```python
from build123d import *

# Parameters (mm, degrees)
SKETCH1_W           = 50
SKETCH1_H           = 50
BOSS_EXTRUDE1_DEPTH = 5
SKETCH2_W           = 50
SKETCH2_H           = 5
BOSS_EXTRUDE2_DEPTH = 50
SKETCH3_R           = 2.6
CUT_EXTRUDE1_DEPTH  = 50
CHAMFER1_SIZE       = 20
SKETCH4_R           = 2.6
CUT_EXTRUDE2_DEPTH  = 50
CHAMFER2_SIZE       = 20
CHAMFER3_SIZE       = 2
CHAMFER4_SIZE       = 2


with BuildPart() as part:
    # Sketch1 → Boss-Extrude1 (new body)
    with BuildSketch(Plane(origin=(0, 0, 0), x_dir=(1, 0, 0), z_dir=(0, 1, 0))):
        Rectangle(SKETCH1_W, SKETCH1_H)
    extrude(amount=BOSS_EXTRUDE1_DEPTH)

    # Sketch2 → Boss-Extrude2 (add)
    with BuildSketch(Plane(origin=(0, 5, 0), x_dir=(1, 0, 0), z_dir=(0, 1, 0))):
        with Locations((0, 22.5)):
            Rectangle(SKETCH2_W, SKETCH2_H)
    extrude(amount=BOSS_EXTRUDE2_DEPTH)

    # Sketch3 → Cut-Extrude1 (cut)
    with BuildSketch(Plane.XY.offset(-20)):
        with Locations((0, 30)):
            Circle(SKETCH3_R)
    extrude(amount=-CUT_EXTRUDE1_DEPTH, mode=Mode.SUBTRACT)

    # Chamfer1
    chamfer1_edges = [part.edges().sort_by_distance(p)[0] for p in [
        (25, 55, -22.5),
        (-25, 55, -22.5),
    ]]
    chamfer(chamfer1_edges, length=CHAMFER1_SIZE)

    # Sketch4 → Cut-Extrude2 (cut)
    with BuildSketch(Plane(origin=(0, 5, 0), x_dir=(1, 0, 0), z_dir=(0, 1, 0))):
        with Locations(Location((0, -5, 0), (0, 0, 270))):
            Circle(SKETCH4_R)
    extrude(amount=-CUT_EXTRUDE2_DEPTH, mode=Mode.SUBTRACT)

    # Chamfer2
    chamfer2_edges = [part.edges().sort_by_distance(p)[0] for p in [
        (25, 2.5, 25),
        (-25, 2.5, 25),
    ]]
    chamfer(chamfer2_edges, length=CHAMFER2_SIZE)

    # Chamfer3
    chamfer3_edges = [part.edges().sort_by_distance(p)[0] for p in [
        (0, 0, -25),
    ]]
    chamfer(chamfer3_edges, length=CHAMFER3_SIZE)

    # Chamfer4
    # the kernel refuses this chamfer: 2 mm, written as the material it takes off along each edge
    with BuildSketch(Plane(origin=(25, 0, -28.143365976), x_dir=(-0.9996219169112968, -0.02749587661058639, 0), z_dir=(0, 0, 1))) as chamfer4_piece_1:
        Polygon((CHAMFER4_SIZE * 0.999621916911, -CHAMFER4_SIZE * 0.0274958766106), (-CHAMFER4_SIZE * 0.0274958766106, -CHAMFER4_SIZE * 0.999621916911), (0, 0), align=None)
    extrude(amount=38.286731952, mode=Mode.SUBTRACT)
    with BuildSketch(Plane(origin=(28.63690896, 0, 1.36309104), x_dir=(-0.7068394360706735, -0.027495876610586382, -0.7068394360706735), z_dir=(-0.7071067811865475, 0, 0.7071067811865476)), Plane(origin=(1.36309104, 58.63690896, -25), x_dir=(-0.7068394360706736, -0.7068394360706737, -0.027495876610585657), z_dir=(0.7071067811865476, -0.7071067811865476, 0)), Plane(origin=(-28.63690896, 31.36309104, -25), x_dir=(0.7068394360706735, -0.7068394360706735, -0.02749587661058563), z_dir=(0.7071067811865476, 0.7071067811865476, 0))) as chamfer4_piece_2:
        Polygon((CHAMFER4_SIZE * 0.999621916911, -CHAMFER4_SIZE * 0.0274958766106), (-CHAMFER4_SIZE * 0.0274958766106, -CHAMFER4_SIZE * 0.999621916911), (0, 0), align=None)
    extrude(amount=38.571003199, mode=Mode.SUBTRACT)
    with BuildSketch(Plane(origin=(10.143365976, 0, 25), x_dir=(0, -0.02749587661058639, -0.9996219169112968), z_dir=(-1, 0, 0))) as chamfer4_piece_3:
        Polygon((CHAMFER4_SIZE * 0.999621916911, -CHAMFER4_SIZE * 0.0274958766106), (-CHAMFER4_SIZE * 0.0274958766106, -CHAMFER4_SIZE * 0.999621916911), (0, 0), align=None)
    extrude(amount=20.286731952, mode=Mode.SUBTRACT)
    with BuildSketch(Plane(origin=(-28.63690896, 0, 1.36309104), x_dir=(0.7068394360706733, -0.027495876610586358, -0.7068394360706735), z_dir=(0.7071067811865476, 0, 0.7071067811865475))) as chamfer4_piece_4:
        Polygon((CHAMFER4_SIZE * 0.999621916911, CHAMFER4_SIZE * 0.0274958766106), (-CHAMFER4_SIZE * 0.0274958766106, CHAMFER4_SIZE * 0.999621916911), (0, 0), align=None)
    extrude(amount=38.571003199, mode=Mode.SUBTRACT)
    with BuildSketch(Plane(origin=(-25, 0, 10.143365976), x_dir=(-0.02749587661058563, 0.9996219169112968, 0), z_dir=(0, 0, -1))) as chamfer4_piece_5:
        Polygon((CHAMFER4_SIZE * 0.999621916911, CHAMFER4_SIZE * 0.0274958766106), (-CHAMFER4_SIZE * 0.0274958766106, CHAMFER4_SIZE * 0.999621916911), (0, 0), align=None)
    extrude(amount=38.286731952, mode=Mode.SUBTRACT)
    with BuildSketch(Plane(origin=(25, 40.143365976, -25), x_dir=(-0.9996219169112968, 0, -0.027495876610585647), z_dir=(0, -1, 0))) as chamfer4_piece_6:
        Polygon((CHAMFER4_SIZE * 0.999621916911, -CHAMFER4_SIZE * 0.0274958766106), (-CHAMFER4_SIZE * 0.0274958766106, -CHAMFER4_SIZE * 0.999621916911), (0, 0), align=None)
    extrude(amount=43.286731952, mode=Mode.SUBTRACT)
    with BuildSketch(Plane(origin=(10.143365976, 55, -25), x_dir=(0, -0.9996219169112968, -0.027495876610585647), z_dir=(-1, 0, 0))) as chamfer4_piece_7:
        Polygon((CHAMFER4_SIZE * 0.999621916911, CHAMFER4_SIZE * 0.0274958766106), (-CHAMFER4_SIZE * 0.0274958766106, CHAMFER4_SIZE * 0.999621916911), (0, 0), align=None)
    extrude(amount=20.286731952, mode=Mode.SUBTRACT)
    with BuildSketch(Plane(origin=(-25, -3.143365976, -25), x_dir=(-0.027495876610585647, 0, 0.9996219169112968), z_dir=(0, 1, 0))) as chamfer4_piece_8:
        Polygon((CHAMFER4_SIZE * 0.999621916911, CHAMFER4_SIZE * 0.0274958766106), (-CHAMFER4_SIZE * 0.0274958766106, CHAMFER4_SIZE * 0.999621916911), (0, 0), align=None)
    extrude(amount=43.286731952, mode=Mode.SUBTRACT)


solid = part.part
```
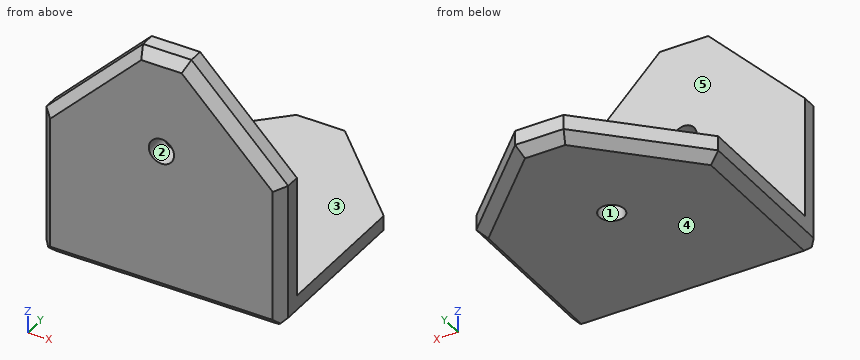
Here's how the part is built. I have some questions about the finished solid (model axes, mm). Face numbers are marked on the shaded views. A direction names the side the tool comes from. Coordinates: 2 decimals unless noted, no trailing zeros. Loops run counter-clockwise (first coordinate to the right, second up) from the corner with the lowest first, then second, coordinate; pieces in that order, holes last. Notation, with made-up numbers: M 17.25,-25 L 63.25,-25 A20 cw 63.25,2 Z; hole C 80.25,8 d4. An arc over 180 degrees is marked long. One line per item, written item: value.
1. Imagine slicing it at C-C (z = -21). List the corners of the cut face in (x, y) for me, and give its area (3 significant figures).
Geometry says:
outline: M -25,2 L -23,0 L 23,0 L 25,2 L 25,35 L 5,55 L -5,55 L -25,35 Z; hole C 0,30 d5.2
area: 2,320 mm2
2. Imagine slicing it at A-A (x = 0). List the corners of the cut face in (y, z) for me, and give its area (3 significant figures).
Geometry says:
outline: M 0,-23 L 2,-25 L 27.4,-25 L 27.4,-20 L 5,-20 L 5,2.4 L 0,2.4 Z; M 0,7.6 L 5,7.6 L 5,25 L 2,25 L 0,23 Z; M 32.6,-25 L 53,-25 L 55,-23 L 55,-20 L 32.6,-20 Z
area: 442 mm2
3. Imagine slicing it at D-D (x = 6.5). List the corners of the cut face in (y, z) for me, and give its area (3 significant figures).
Geometry says:
outline: M 0,-23 L 2,-25 L 50.67,-25 L 53.5,-23 L 53.5,-20 L 5,-20 L 5,23.5 L 2,23.5 L 0,20.67 Z
area: 477 mm2
4. Will these pins go through, and if not, where does the flat tip stop? pin 1 Ø2 at (x, y) = (18, 32.5) entering from +Z; pin 2 Ø12 at (x, y) = (-13, 45.5) entering from -Z; pin 3 Ø10 at (x, z) = (0.5, 19.5) entering from +Y.
Geometry says:
pin 1: stops at z = -20
pin 2: stops at z = -25
pin 3: stops at y = 5
5. Please list where these lines run through material, in increasing order: probe 1 along Y at (x, z) = (0, -21.5); probe 2 along X at (y, z) = (3, 5); probe 3 along Y at (x, z) = (4, 9.5).
Geometry says:
probe 1: y = 0 to 27.4, 32.6 to 55
probe 2: x = -25 to -2.6, 2.6 to 25
probe 3: y = 0 to 5
6. Imagine slicing it at B-B (y = 30). List the corners of the cut face in (x, z) for me.
Geometry says:
outline: M -25,-23 L -23,-25 L -2.6,-25 L -2.6,-20 L -25,-20 Z; M 2.6,-25 L 23,-25 L 25,-23 L 25,-20 L 2.6,-20 Z
7. Thinking about a two-plate mould opening in X: for the marked faces 1, 2 and 3, which applies, +X half, -X half, draft (parallel to the pull), parting line (faces both ways), or undercut?
Geometry says:
face 1: undercut
face 2: undercut
face 3: draft
8. On a 3-axis mill with a long thin cutter (end or side, diameter ignored), from which of +Z, -Z, +X, -X, +Y, -Y can I reach the whole of each face in a straight line? I mean the marked faces 4 and 5. Say none if no direction works.
Geometry says:
face 4: -Z, +X, -X, +Y, -Y
face 5: +Z, +X, -X, +Y
